The listing builds one solid part. Answer for the finished solid, in the listing's coordinates (mm). Face numbers are marked on the shaded views. A direction names the side the tool comes from. Give positions to 0.01 mm unless a question says otherwise; leave off trailing zeros. Loops run counter-clockwise (first coordinate to the right, second up) from the corner with the lowest first, then second, coordinate; pieces in that order, holes last. Notation, with made-up numbers: (-28.5, 21) - (-12.5, 21) arc R15 ccw to (-12.5, 29) - close; hole circle Ø1 at (0.25, 31). An arc over 180 degrees is marked (long way). Write each question's results on one line, items separated by ' | '.
from build123d import *

# Parameters (mm, degrees)
EXTRUDE_1_DEPTH             = 3
SKETCH_3_R                  = 11
CUT_EXTRUDE_1_DEPTH         = 2
CUT_EXTRUDE_2_DEPTH         = 20
CUT_EXTRUDE_2_DEPTH_BACK    = 42.593268686
SKETCH_1_R                  = 3
SKETCH_1_R_2                = 2
EXTRUDE_2_DEPTH             = 3
SKETCH_5_R                  = 3.5
CUT_EXTRUDE_3_DEPTH         = 58.282196187
SKETCH_8_W                  = 20
SKETCH_8_H                  = 22
EXTRUDE_4_DEPTH             = 3
EXTRUDE_5_REACH             = 57.256
EXTRUDE_5_DIRECTION_2_REACH = 57.256
SKETCH_11_W                 = 5
SKETCH_11_H                 = 5
EXTRUDE_6_DEPTH             = 15
EXTRUDE_6_2_DEPTH           = 15
SKETCH_13_W                 = 2
SKETCH_13_H                 = 22
EXTRUDE_7_DEPTH             = 33
SKETCH_15_W                 = 2
SKETCH_15_H                 = 5
EXTRUDE_8_DEPTH             = 28
SKETCH_14_R                 = 1.75
CUT_EXTRUDE_4_DEPTH         = 69.163406605
SKETCH_16_W                 = 2
SKETCH_16_H                 = 7
EXTRUDE_9_DEPTH             = 6.5
SKETCH_17_W                 = 2
SKETCH_17_H                 = 7
EXTRUDE_10_DEPTH            = 15
SKETCH_18_W                 = 2
SKETCH_18_H                 = 7
EXTRUDE_11_DEPTH            = 21.5
SKETCH_19_R                 = 2.5
EXTRUDE_12_DEPTH            = 4
CUT_EXTRUDE_5_REACH         = 66.773
SKETCH_20_W                 = 14
SKETCH_20_H                 = 20
SKETCH_21_W                 = 25
SKETCH_21_H                 = 14
CUT_EXTRUDE_6_DEPTH         = 72.045759902
CHAMFER_1_SIZE              = 4
FILLET_1_R                  = 4
FILLET_2_R                  = 2
FILLET_3_R                  = 2
FILLET_4_R                  = 1


with BuildPart() as part:
    # Sketch 2 → Extrude 1 (new body)
    with BuildSketch(Plane(origin=(0, 0, 0), x_dir=(1, 0, 0), z_dir=(0, 1, 0))):
        with BuildLine():
            Line((0, 11), (40, 11))
            Line((40, 11), (40, -11))
            Line((40, -11), (0, -11))
            ThreePointArc((0, -11), (-11, 0), (0, 11))
        make_face()
    extrude(amount=EXTRUDE_1_DEPTH)

    # Sketch 3 → Cut-Extrude 1 (cut)
    with BuildSketch(Plane(origin=(0, 0, 0), x_dir=(-1, 0, 0), z_dir=(0, -1, 0))):
        Circle(SKETCH_3_R)
    extrude(amount=-CUT_EXTRUDE_1_DEPTH, mode=Mode.SUBTRACT)

    # Sketch 1 → Cut-Extrude 2 (cut, two sides: drawn at the far end of the back side and taken through both)
    with BuildSketch(Plane(origin=(0, 0, 0), x_dir=(1, 0, 0), z_dir=(0, 1, 0)).offset(-CUT_EXTRUDE_2_DEPTH_BACK)):
        with Locations(Location((0, 0, 0), (0, 0, 90))):
            Circle(SKETCH_1_R)
        with Locations(Location((-7, 0, 0), (0, 0, 90))):
            Circle(SKETCH_1_R_2)
        with Locations(Location((0, 7, 0), (0, 0, 90))):
            Circle(SKETCH_1_R_2)
        with Locations(Location((7, 0, 0), (0, 0, 90))):
            Circle(SKETCH_1_R_2)
        with Locations(Location((0, -7, 0), (0, 0, 90))):
            Circle(SKETCH_1_R_2)
    extrude(amount=CUT_EXTRUDE_2_DEPTH + CUT_EXTRUDE_2_DEPTH_BACK, mode=Mode.SUBTRACT)


with BuildPart() as body_2:
    # Sketch 4 → Extrude 2 (new body)
    with BuildSketch(Plane(origin=(0, -33.5, 0), x_dir=(-1, 0, 0), z_dir=(0, -1, 0))):
        with BuildLine():
            Line((0, 11), (-10, 11))
            Line((-10, 11), (-10, -11))
            Line((-10, -11), (0, -11))
            ThreePointArc((0, -11), (11, 0), (0, 11))
        make_face()
    extrude(amount=EXTRUDE_2_DEPTH)


with BuildPart() as cut_extrude_3_tool:
    # Sketch 5 → Cut-Extrude 3 (new, through all)
    with BuildSketch(Plane(origin=(0, -36.5, 0), x_dir=(-1, 0, 0), z_dir=(0, -1, 0))):
        with Locations(Location((0, 0, 0), (0, 0, 180))):
            Circle(SKETCH_5_R)
    extrude(amount=-CUT_EXTRUDE_3_DEPTH)


with BuildPart() as part_1:
    add(part.part)

    # Cut-Extrude 3: cut by cut_extrude_3_tool
    add(cut_extrude_3_tool.part, mode=Mode.SUBTRACT)



with BuildPart() as body_2_1:
    add(body_2.part)

    # Cut-Extrude 3: cut by cut_extrude_3_tool
    add(cut_extrude_3_tool.part, mode=Mode.SUBTRACT)


with BuildPart() as body_3:
    # Sketch 8 → Extrude 4 (new body)
    with BuildSketch(Plane(origin=(0, -27, 0), x_dir=(-1, 0, 0), z_dir=(0, -1, 0))):
        with Locations((-30, 0)):
            Rectangle(SKETCH_8_W, SKETCH_8_H)
    extrude(amount=EXTRUDE_4_DEPTH)

    # Extrude 5: up to this face of the body (flat: up to its plane)
    extrude_5_end = Plane(body_3.part.faces().sort_by_distance((30, -28.5, 11))[0])
    # Sketch 10 → Extrude 5 (add, up to the picked face)
    with BuildSketch(Plane.XY, mode=Mode.PRIVATE) as extrude_5_sk1:
        Polygon((10, -36.5), (20, -30), (20, -27), (10, -33.5), align=None)
    extrude_5_tool1 = split(extrude(extrude_5_sk1.sketch, amount=EXTRUDE_5_REACH, mode=Mode.PRIVATE), bisect_by=extrude_5_end, keep=Keep.BOTH, mode=Mode.PRIVATE)

    add(body_2_1.part)  # Extrude 5 merges body 2
    add(extrude_5_tool1.solids().sort_by(Axis((15, -31.75, 0), (0, 0, 1)))[0])

    # Extrude 5 direction 2: up to this face of the body (flat: up to its plane)
    extrude_5_direction_2_end = Plane(body_3.part.faces().sort_by_distance((30, -28.5, -11))[0])
    # Sketch 10 → Extrude 5 direction 2 (add, up to the picked face)
    with BuildSketch(Plane.XY, mode=Mode.PRIVATE) as extrude_5_direction_2_sk1:
        Polygon((10, -36.5), (20, -30), (20, -27), (10, -33.5), align=None)
    extrude_5_direction_2_tool1 = split(extrude(extrude_5_direction_2_sk1.sketch, amount=-EXTRUDE_5_DIRECTION_2_REACH, mode=Mode.PRIVATE), bisect_by=extrude_5_direction_2_end, keep=Keep.BOTH, mode=Mode.PRIVATE)
    add(extrude_5_direction_2_tool1.solids().sort_by(Axis((15, -31.75, 0), (0, 0, -1)))[0])


with BuildPart() as body_3_2:
    # Sketch 11 → Extrude 6 (new body)
    with BuildSketch(Plane(origin=(40, 0, 0), x_dir=(0, 0, -1), z_dir=(1, 0, 0))):
        with Locations((8.5, 0.5)):
            Rectangle(SKETCH_11_W, SKETCH_11_H)
    extrude(amount=EXTRUDE_6_DEPTH)


with BuildPart() as body_4:
    # Sketch 11 → Extrude 6 2 (new body)
    with BuildSketch(Plane(origin=(40, 0, 0), x_dir=(0, 0, -1), z_dir=(1, 0, 0))):
        with Locations((8.5, -27.5)):
            Rectangle(SKETCH_11_W, SKETCH_11_H)
    extrude(amount=EXTRUDE_6_2_DEPTH)


with BuildPart() as part_2:
    add(part_1.part)

    add(body_3.part)  # Extrude 7 merges body 3

    add(body_3_2.part)  # Extrude 7 merges body 3 2

    add(body_4.part)  # Extrude 7 merges body 4
    # Sketch 13 → Extrude 7 (add)
    with BuildSketch(Plane(origin=(0, 3, 0), x_dir=(1, 0, 0), z_dir=(0, 1, 0))):
        with Locations((39, 0)):
            Rectangle(SKETCH_13_W, SKETCH_13_H)
    extrude(amount=-EXTRUDE_7_DEPTH)

    # Sketch 15 → Extrude 8 (add)
    with BuildSketch(Plane.XZ.offset(2)):
        with Locations((54, -8.5)):
            Rectangle(SKETCH_15_W, SKETCH_15_H)
    extrude(amount=EXTRUDE_8_DEPTH)

    # Sketch 14 → Cut-Extrude 4 (cut, through all)
    with BuildSketch(Plane.XY.offset(-6)):
        with Locations((46.5, 0.25)):
            Circle(SKETCH_14_R)
        with Locations(Location((46.5, -27.25, 0), (0, 0, 180))):
            Circle(SKETCH_14_R)
    extrude(amount=-CUT_EXTRUDE_4_DEPTH, mode=Mode.SUBTRACT)

    # Sketch 16 → Extrude 9 (add)
    with BuildSketch(Plane.XY.offset(11)):
        with Locations((39, -18.95)):
            Rectangle(SKETCH_16_W, SKETCH_16_H)
    extrude(amount=EXTRUDE_9_DEPTH)

    # Sketch 17 → Extrude 10 (add)
    with BuildSketch(Plane(origin=(40, 0, 0), x_dir=(0, 0, -1), z_dir=(1, 0, 0))):
        with Locations((-16.5, -18.95)):
            Rectangle(SKETCH_17_W, SKETCH_17_H)
    extrude(amount=EXTRUDE_10_DEPTH)

    # Sketch 18 → Extrude 11 (add)
    with BuildSketch(Plane(origin=(0, 0, 15.5), x_dir=(-1, 0, 0), z_dir=(0, 0, -1))):
        with Locations((-54, -18.95)):
            Rectangle(SKETCH_18_W, SKETCH_18_H)
    extrude(amount=EXTRUDE_11_DEPTH)

    # Sketch 19 → Extrude 12 (add)
    with BuildSketch(Plane.XY.offset(17.5)):
        with Locations((46.5, -18.95)):
            Circle(SKETCH_19_R)
    extrude(amount=EXTRUDE_12_DEPTH)

    # Sketch 20 → Cut-Extrude 5 (cut, up to next)
    with BuildSketch(Plane.ZY.offset(-38), mode=Mode.PRIVATE) as cut_extrude_5_sk1:
        with Locations((0, -13.5)):
            Rectangle(SKETCH_20_W, SKETCH_20_H)
    cut_extrude_5_tool1 = extrude(cut_extrude_5_sk1.sketch, amount=-CUT_EXTRUDE_5_REACH, mode=Mode.PRIVATE) & part_2.part
    add(cut_extrude_5_tool1.solids().sort_by_distance((38, -13.5, 0))[0], mode=Mode.SUBTRACT)

    # Sketch 21 → Cut-Extrude 6 (cut, through all)
    with BuildSketch(Plane(origin=(0, 3, 0), x_dir=(1, 0, 0), z_dir=(0, 1, 0))):
        with Locations((24, 0)):
            Rectangle(SKETCH_21_W, SKETCH_21_H)
    extrude(amount=-CUT_EXTRUDE_6_DEPTH, mode=Mode.SUBTRACT)

    # Chamfer 1
    # the kernel refuses this chamfer: 4 mm, written as the material it adds along each edge
    with BuildSketch(Plane(origin=(38, -27, -11), x_dir=(-0.999621916911297, -0.027495876610579655, 0), z_dir=(0, 0, 1))) as chamfer_1_piece_1_section:
        Polygon((CHAMFER_1_SIZE * 0.999621916911, -CHAMFER_1_SIZE * 0.0274958766106), (-CHAMFER_1_SIZE * 0.0274958766106, -CHAMFER_1_SIZE * 0.999621916911), (0, 0), align=None)
    chamfer_1_piece_1 = extrude(amount=32.286731952, mode=Mode.PRIVATE)
    chamfer_1_piece_1 = split(chamfer_1_piece_1, bisect_by=Plane(origin=(35.666666667, -26.166666667, -7), z_dir=(0, 0, -1)), keep=Keep.TOP, mode=Mode.PRIVATE)
    add(chamfer_1_piece_1)
    with BuildSketch(Plane(origin=(38, -27, -11), x_dir=(-0.999621916911297, -0.027495876610579655, 0), z_dir=(0, 0, 1))) as chamfer_1_piece_2_section:
        Polygon((CHAMFER_1_SIZE * 0.999621916911, -CHAMFER_1_SIZE * 0.0274958766106), (-CHAMFER_1_SIZE * 0.0274958766106, -CHAMFER_1_SIZE * 0.999621916911), (0, 0), align=None)
    chamfer_1_piece_2 = extrude(amount=22, mode=Mode.PRIVATE)
    chamfer_1_piece_2 = split(chamfer_1_piece_2, bisect_by=Plane(origin=(36.5, -25.399122807, 0), z_dir=(1, 0, 0)), keep=Keep.TOP, mode=Mode.PRIVATE)
    chamfer_1_piece_2 = split(chamfer_1_piece_2, bisect_by=Plane(origin=(37.293859649, -23.5, 0), z_dir=(0, -1, 0)), keep=Keep.TOP, mode=Mode.PRIVATE)
    add(chamfer_1_piece_2)
    with BuildSketch(Plane(origin=(38, -27, -21.286731952), x_dir=(-0.999621916911297, -0.02749587661057961, 0), z_dir=(0, 0, 1))) as chamfer_1_piece_3_section:
        Polygon((CHAMFER_1_SIZE * 0.999621916911, -CHAMFER_1_SIZE * 0.0274958766106), (-CHAMFER_1_SIZE * 0.0274958766106, -CHAMFER_1_SIZE * 0.999621916911), (0, 0), align=None)
    chamfer_1_piece_3 = extrude(amount=32.286731952, mode=Mode.PRIVATE)
    chamfer_1_piece_3 = split(chamfer_1_piece_3, bisect_by=Plane(origin=(35.666666667, -26.166666667, 7), z_dir=(0, 0, 1)), keep=Keep.TOP, mode=Mode.PRIVATE)
    add(chamfer_1_piece_3)
    with BuildSketch(Plane(origin=(38, 0, 11), x_dir=(0.02749587661058563, -0.9996219169112968, 0), z_dir=(0, 0, -1))) as chamfer_1_piece_4_section:
        Polygon((CHAMFER_1_SIZE * 0.999621916911, CHAMFER_1_SIZE * 0.0274958766106), (-CHAMFER_1_SIZE * 0.0274958766106, CHAMFER_1_SIZE * 0.999621916911), (0, 0), align=None)
    chamfer_1_piece_4 = extrude(amount=32.286731952, mode=Mode.PRIVATE)
    chamfer_1_piece_4 = split(chamfer_1_piece_4, bisect_by=Plane(origin=(37.833333333, -3.666666667, 7), z_dir=(0, 0, 1)), keep=Keep.TOP, mode=Mode.PRIVATE)
    add(chamfer_1_piece_4)
    with BuildSketch(Plane(origin=(38, 0, 21.286731952), x_dir=(0.02749587661058563, -0.9996219169112968, 0), z_dir=(0, 0, -1))) as chamfer_1_piece_5_section:
        Polygon((CHAMFER_1_SIZE * 0.999621916911, CHAMFER_1_SIZE * 0.0274958766106), (-CHAMFER_1_SIZE * 0.0274958766106, CHAMFER_1_SIZE * 0.999621916911), (0, 0), align=None)
    chamfer_1_piece_5 = extrude(amount=32.286731952, mode=Mode.PRIVATE)
    chamfer_1_piece_5 = split(chamfer_1_piece_5, bisect_by=Plane(origin=(37.293859649, -1.600877193, 7), z_dir=(0, 0, -1)), keep=Keep.TOP, mode=Mode.PRIVATE)
    chamfer_1_piece_5 = split(chamfer_1_piece_5, bisect_by=Plane(origin=(37.293859649, -3.5, 0), z_dir=(0, 1, 0)), keep=Keep.TOP, mode=Mode.PRIVATE)
    chamfer_1_piece_5 = split(chamfer_1_piece_5, bisect_by=Plane(origin=(36.5, -1.600877193, 0), z_dir=(1, 0, 0)), keep=Keep.TOP, mode=Mode.PRIVATE)
    add(chamfer_1_piece_5)
    with BuildSketch(Plane(origin=(38, 0, 21.286731952), x_dir=(0.02749587661058563, -0.9996219169112968, 0), z_dir=(0, 0, -1))) as chamfer_1_piece_6_section:
        Polygon((CHAMFER_1_SIZE * 0.999621916911, CHAMFER_1_SIZE * 0.0274958766106), (-CHAMFER_1_SIZE * 0.0274958766106, CHAMFER_1_SIZE * 0.999621916911), (0, 0), align=None)
    chamfer_1_piece_6 = extrude(amount=32.286731952, mode=Mode.PRIVATE)
    chamfer_1_piece_6 = split(chamfer_1_piece_6, bisect_by=Plane(origin=(37.833333333, -3.666666667, -7), z_dir=(0, 0, -1)), keep=Keep.TOP, mode=Mode.PRIVATE)
    add(chamfer_1_piece_6)

    # Fillet 1
    fillet_1_edges = [part_2.edges().sort_by_distance(p)[0] for p in [
        (20, -30, -9),
        (10, -33.5, 0),
        (20, -30, 9),
    ]]
    fillet(fillet_1_edges, radius=FILLET_1_R)

    # Fillet 2
    fillet_2_edges = [part_2.edges().sort_by_distance(p)[0] for p in [
        (55, 3, -8.5),
        (55, -30, -8.5),
    ]]
    fillet(fillet_2_edges, radius=FILLET_2_R)

    # Fillet 3
    fillet_3_edges = [part_2.edges().sort_by_distance(p)[0] for p in [
        (39, -22.45, 11),
        (39, -15.45, 11),
        (54, -15.45, -6),
        (54, -22.45, -6),
    ]]
    fillet(fillet_3_edges, radius=FILLET_3_R)

    # Fillet 4
    fillet_4_edges = [part_2.edges().sort_by_distance(p)[0] for p in [
        (38, -18.95, 17.5),
        (55, -18.95, 17.5),
    ]]
    fillet(fillet_4_edges, radius=FILLET_4_R)


solid = part_2.part
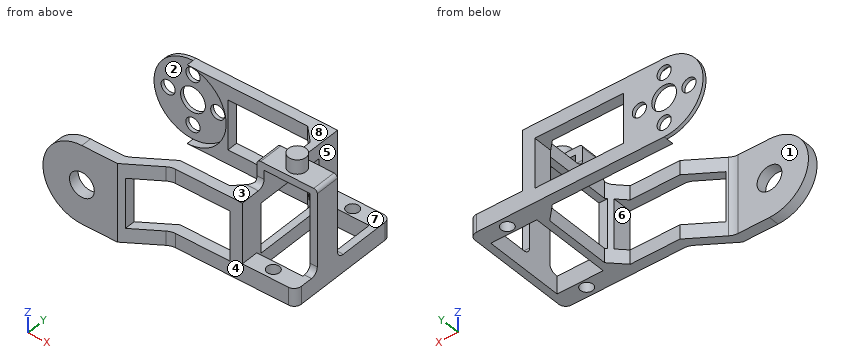
Item 1: Flat-ended cylindrical pins translate along their axes: P1, Ø8, axis at x = 19.5, y = -2, coming from the -Z side; P2, Ø1.2, axis at x = 39.5, y = -16.5, coming from the +Z side; P3, Ø1, axis at x = -4.5, z = 12, coming from the +Y side; P4, Ø6, axis at y = 0, z = -3.5, coming from the -X side. Find the tip coordinate at first contact, or state that the pin passes through.
Values found:
P1: stops at z = -11 | P2: stops at z = 17.5 | P3: passes through | P4: stops at x = -10.93
Item 2: A cutting plane is placed at D-D, the plane x = -7. Determine the outline of the cut face in (y, z), plus the area to 3 significant figures.
Values found:
outline: (-36.5, -8.49) - (-33.5, -8.49) - (-33.5, 8.49) - (-36.5, 8.49) - close; (2, -8.49) - (3, -8.49) - (3, -2) - (2, -2) - close; (2, 2) - (3, 2) - (3, 8.49) - (2, 8.49) - close | area: 63.9 mm²
Item 3: A cutting plane is placed at B-B, the plane x = 33. Determine the outline of the cut face in (y, z).
Values found:
outline: (-30, -11) - (-27, -11) - (-27, -7) - (-30, -7) - close; (-30, 7) - (-27, 7) - (-27, 11) - (-30, 11) - close; (0, -11) - (3, -11) - (3, -7) - (0, -7) - close; (0, 7) - (3, 7) - (3, 11) - (0, 11) - close
Item 4: Find the intervals of material crossed by line 1 along Y through (x, z) = (5.5, -4); line 2 along X through (y, z) = (-17.5, 12.5); line 3 along X through (y, z) = (-27.25, -9.25), in increasing order. Write a range as [from, to].
Values found:
line 1: y = [-36.5, -33.5], [2, 3] | line 2: x = [38, 40], [53, 55] | line 3: x = [19.62, 44.75], [48.25, 55]
Item 5: For the marked faces 5, 6, 7 and 8, determine the directions among +Z, -Z, +X, -X, +Y, -Y from which every point of the face is accessible in a straight line to the end or side of a thin tool.
Values found:
face 5: none | face 6: -X, +Y, -Y | face 7: +Z, +X, +Y | face 8: +Z, +X, -X, +Y
Item 6: For a pull along Y with two mould halves and no side action, classify the marked faces 1, 2, 3 and 4 as released by +Y, released by -Y, zero draft, split by the parting line, or undercut.
Values found:
face 1: undercut | face 2: undercut | face 3: zero draft | face 4: released by -Y
Item 7: A cutting plane is placed at C-C, the plane z = 0. Count the separate pieces of the cut face and the enclosed holes in it, plus the area to 3 significant figures.
Values found:
separate pieces: 9 | enclosed holes: 0 | area: 114 mm²
Item 8: A cutting plane is placed at A-A, the plane y = -18.95. Determine the outline of the cut face in (x, z).
Values found:
outline: (38, -11) - (40, -11) - (40, -7) - (38, -7) - close; (38, 7) - (40, 7) - (40, 15.5) - (53, 15.5) - (53, -11) - (55, -11) - (55, 16.5) arc R1 ccw to (54, 17.5) - (49, 17.5) - (49, 21.5) - (44, 21.5) - (44, 17.5) - (39, 17.5) arc R1 ccw to (38, 16.5) - close
